The listing builds one solid part. Answer for the finished solid, in the listing's coordinates (mm). Face numbers are marked on the shaded views. A direction names the side the tool comes from. Give positions to 0.01 mm unless a question says otherwise; leave off trailing zeros. Order: outer loops, then holes, each group sorted by start corner. A loop starts at its lowest first (then second) coordinate and runs counter-clockwise, first axis right, second up. Notation, with made-up numbers: (26.5, 63.5) - (54.5, 63.5) arc R16 cw to (54.5, 94.5) - close; hole circle Ø11 at (24.5, -7.5). An arc over 180 degrees is marked (long way). Answer as a JSON object with one key per item and string values. Group by question number.
Q1. Given pin 1 (1.8 mm diameter, centred on y = -6.5, z = 27, fed in from +X); pin 2 (1.5 mm diameter, centred on x = -13.5, z = 78.5, fed in from +Y); pin 3 (1.5 mm diameter, centred on y = -7.5, z = 10.5, fed in from +X), each flat-ended and moving along its own axis, determine where each tip first touches the part or whether it passes through.
Q2. The mould has two halves that part along Y. Classify the marked faces 3, 4 and 5: released by +Y, released by -Y, zero draft, split by the parting line, or undercut.
Q3. Consider line 1 (Y direction, x = 9, z = 46); line 2 (X direction, y = -7.5, z = 78.5); line 3 (X direction, y = -6, z = 14.5). Determine where each line is inside the solid, lowest interval first.
Q4. For the marked faces 1 and 2, determine the directions among +Z, -Z, +X, -X, +Y, -Y from which every point of the face is accessible in a straight line to the end or side of a thin tool.
Q5. A cutting plane is placed at A-A, the plane y = -16. Give the vertices of the cut face in (x, z).
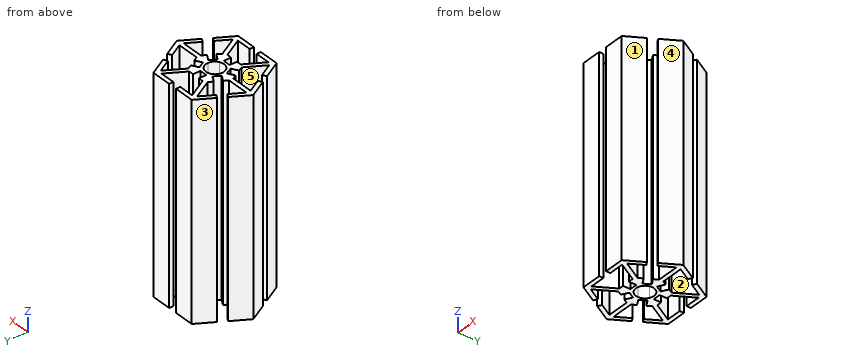
from build123d import *

# Parameters (mm, degrees)
F1_DEPTH = 100


with BuildPart() as f1:
    # F0 (on Top) → F1 (new body)
    with BuildSketch(Plane.XY):
        Polygon((16.270508, 11.818653), (11.547005, 20), (2.1, 20), (2.1, 18), (9.237604, 18), (4.041452, 9), (1.75, 9), (1.75, 5.5), (-1.75, 5.5), (-1.75, 9), (-4.041452, 9), (-9.237604, 18), (-2.1, 18), (-2.1, 20), (-11.547005, 20), (-16.270508, 11.818653), (-14.538457, 10.818653), (-10.969655, 17), (-5.773503, 8), (-6.919229, 6.015544), (-3.88814, 4.265544), (-5.63814, 1.234456), (-8.669229, 2.984456), (-9.814955, 1), (-20.207259, 1), (-16.638457, 7.181347), (-18.370508, 8.181347), (-23.094011, 0), (-18.370508, -8.181347), (-16.638457, -7.181347), (-20.207259, -1), (-9.814955, -1), (-8.669229, -2.984456), (-5.63814, -1.234456), (-3.88814, -4.265544), (-6.919229, -6.015544), (-5.773503, -8), (-10.969655, -17), (-14.538457, -10.818653), (-16.270508, -11.818653), (-11.547005, -20), (-2.1, -20), (-2.1, -18), (-9.237604, -18), (-4.041452, -9), (-1.75, -9), (-1.75, -5.5), (1.75, -5.5), (1.75, -9), (4.041452, -9), (9.237604, -18), (2.1, -18), (2.1, -20), (11.547005, -20), (16.270508, -11.818653), (14.538457, -10.818653), (10.969655, -17), (5.773503, -8), (6.919229, -6.015544), (3.88814, -4.265544), (5.63814, -1.234456), (8.669229, -2.984456), (9.814955, -1), (20.207259, -1), (16.638457, -7.181347), (18.370508, -8.181347), (23.094011, 0), (18.370508, 8.181347), (16.638457, 7.181347), (20.207259, 1), (9.814955, 1), (8.669229, 2.984456), (5.63814, 1.234456), (3.88814, 4.265544), (6.919229, 6.015544), (5.773503, 8), (10.969655, 17), (14.538457, 10.818653), align=None)
        with BuildLine():
            ThreePointArc((-2.125, 3.680608), (0, 4.25), (2.125, 3.680608))
            ThreePointArc((2.125, 3.680608), (3.680608, 2.125), (4.25, 0))
            ThreePointArc((4.25, 0), (3.680608, -2.125), (2.125, -3.680608))
            ThreePointArc((2.125, -3.680608), (0, -4.25), (-2.125, -3.680608))
            ThreePointArc((-2.125, -3.680608), (-3.680608, -2.125), (-4.25, 0))
            ThreePointArc((-4.25, 0), (-3.680608, 2.125), (-2.125, 3.680608))
        make_face(mode=Mode.SUBTRACT)
    extrude(amount=F1_DEPTH)


solid = f1.part
Reply:
{
 "1": {"pin 1": "stops at x = 19.86", "pin 2": "stops at y = 17.92", "pin 3": "stops at x = 19.2"},
 "2": {"face 3": "released by +Y", "face 4": "released by -Y", "face 5": "undercut"},
 "3": {"line 1": "y = -20 to -18, -17.59 to -13.59, -2.41 to 2.41, 13.59 to 17.59, 18 to 20", "line 2": "x = -18.76 to -17.19, -6.06 to -1.75, 1.75 to 6.06, 17.19 to 18.76", "line 3": "x = -19.63 to -17.32, -6.89 to -1.75, 1.75 to 6.89, 17.32 to 19.63"},
 "4": {"face 1": "+Z, -Z, +X, -Y", "face 2": "+Z, -Z"},
 "5": {"outline": "(-13.86, 0) - (-11.55, 0) - (-11.55, 100) - (-13.86, 100) - close; (-10.39, 0) - (-8.08, 0) - (-8.08, 100) - (-10.39, 100) - close; (8.08, 0) - (10.39, 0) - (10.39, 100) - (8.08, 100) - close; (11.55, 0) - (13.86, 0) - (13.86, 100) - (11.55, 100) - close"}
}
